The drawing under review shows one solid part. Ordinate dimensions are in mm from its lowest x, y, z. A direction names the side the tool comes from. Give positions to 0.01 mm unless a question says otherwise; leave off trailing zeros. Order: outer loops, then holes, each group sorted by start corner. A loop starts at its lowest first (then second) coordinate and runs counter-clockwise, first axis right, second up. Notation, with made-up numbers: (61, 13.25) - (113, 13.25) arc R11 cw to (113, 29.25) - close; hole circle Ø4 at (33, 20.5). An arc over 180 degrees is marked (long way). Use CSV: the item, a comma, the result in double quotes.
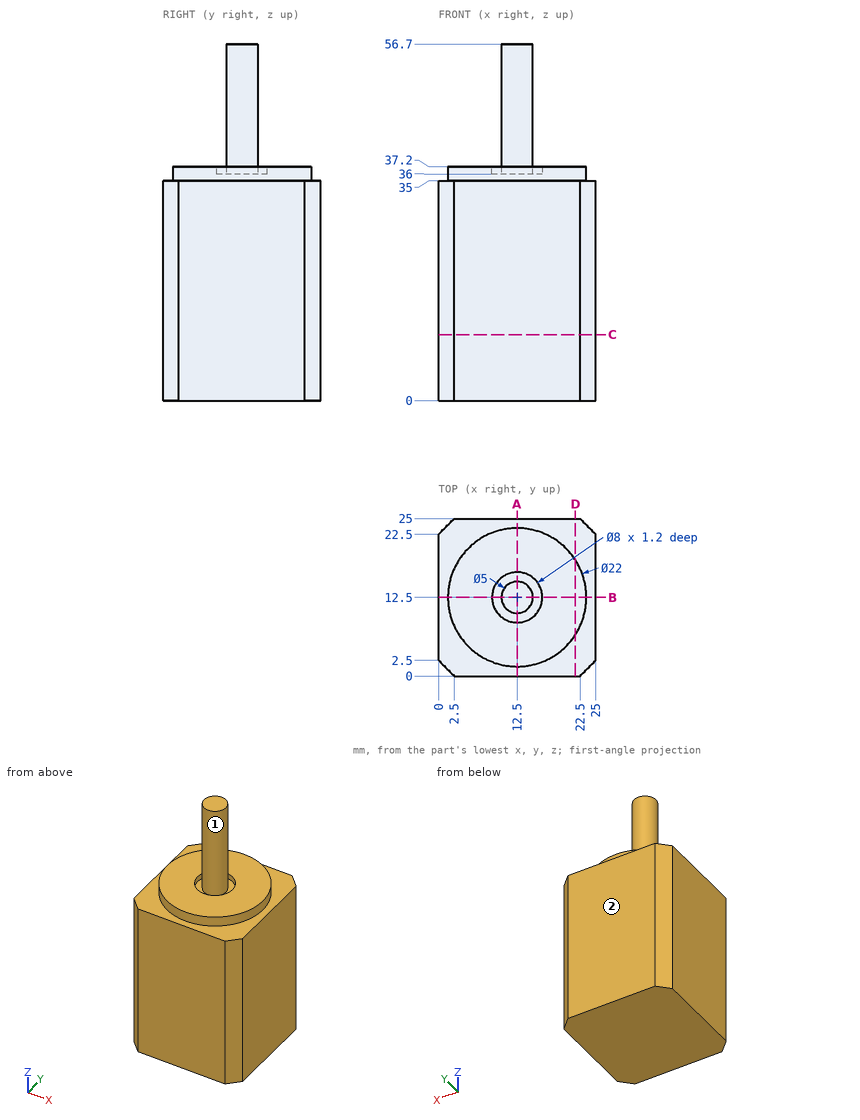
Item 1: Wall thickness on L1, parallel to Y at x = 12.5, z = 36.9; L2, parallel to Z at x = 5, y = 13.75; L3, parallel to Z at x = 14, y = 10: over which ranges is each line inside the solid? List them lowest first.
Results list:
L1,"y = 1.5 to 8.5, 10 to 15, 16.5 to 23.5"
L2,"z = 0 to 37.2"
L3,"z = 0 to 36"
Item 2: Take a section at C-C, the plane z = 10.5. Give the boundary of the cut face in (x, y), and give its area (4 significant figures).
Results list:
outline,"(0, 2.5) - (2.5, 0) - (22.5, 0) - (25, 2.5) - (25, 22.5) - (22.5, 25) - (2.5, 25) - (0, 22.5) - close"
area,"612.5 mm2"
Item 3: Take a section at A-A, the plane x = 12.5. Give the boundary of the cut face in (y, z).
Results list:
outline,"(0, 0) - (25, 0) - (25, 35) - (23.5, 35) - (23.5, 37.2) - (16.5, 37.2) - (16.5, 36) - (15, 36) - (15, 56.7) - (10, 56.7) - (10, 36) - (8.5, 36) - (8.5, 37.2) - (1.5, 37.2) - (1.5, 35) - (0, 35) - close"
Item 4: Clearance check with flat-ended pins moving along their axes: pin 1 (9 mm diameter, centred on x = 12.5, y = 12.5, fed in from -Z); pin 2 (5 mm diameter, centred on y = 4, z = 40.5, fed in from -X); pin 3 (5 mm diameter, centred on y = 11.5, z = 47.5, fed in from -X); pin 4 (1.5 mm diameter, centred on x = 10, z = 44.5, fed in from +Y). State where each tip first meets the part, or that it passes through.
Results list:
pin 1,"stops at z = 0"
pin 2,"passes through"
pin 3,"stops at x = 10"
pin 4,"stops at y = 14.29"
Item 5: Tool access review of the marked faces 1 and 2: name each direction out of +Z, -Z, +X, -X, +Y, -Y from which nothing blocks a thin tool from reaching the whole face with its end or side.
Results list:
face 1,"+Z"
face 2,"+Z, -Z, +X, -X, +Y"
Item 6: Take a section at D-D, the plane x = 21.75. Give the boundary of the cut face in (y, z).
Results list:
outline,"(0, 0) - (25, 0) - (25, 35) - (18.45, 35) - (18.45, 37.2) - (6.55, 37.2) - (6.55, 35) - (0, 35) - close"
